Study the drawing (mm; zero at the part's minimum x, y, z) and answer. Give positions to 0.01 mm unless a question says otherwise; leave off trailing zeros. Loops run counter-clockwise (first coordinate to the right, second up) from the corner with the lowest first, then second, coordinate; pieces in that order, holes last. Notation, with made-up numbers: (62.25, 35.25) - (86.25, 35.25) arc R9 ccw to (86.25, 47.25) - close; hole circle Ø4 at (59.5, -0.75). An arc over 180 degrees is marked (long way). Write item = value, one per line. Start each with the question number.
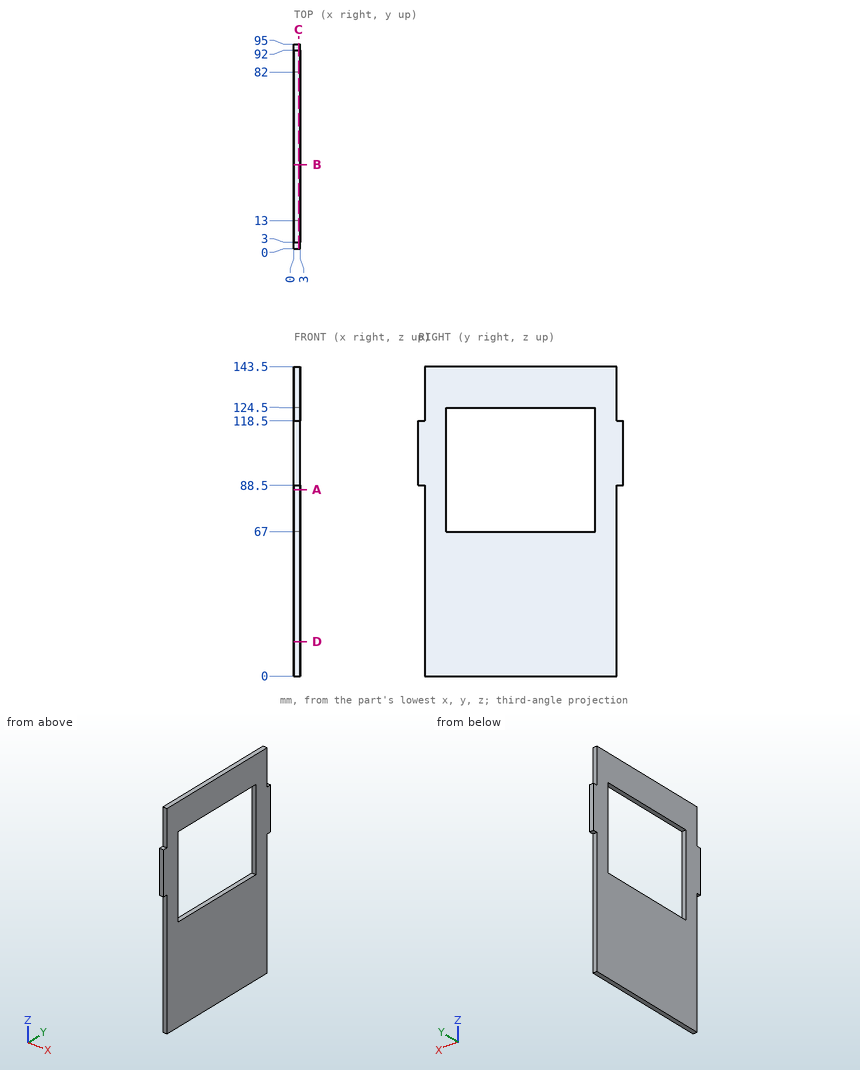
1. A cutting plane is placed at A-A on z = 86.5. Give the vertices of the cut face in (x, y), and give its area (3 significant figures).
2. A cutting plane is placed at D-D on z = 16. Give the vertices of the cut face in (x, y).
3. Consider line 1 along Z through (x, y) = (0.8, 51); line 2 along Y through (x, z) = (2.1, 110.5); line 3 along Y through (x, z) = (2.4, 70.5). Determine where each line is inside the solid, lowest interval first. Write a range as [from, to].
4. A cutting plane is placed at C-C on x = 2.15. Give the vertices of the cut face in (y, z), and give its area (3 significant figures).
5. Given P1, Ø1.5, axis at x = 2, z = 131.5, coming from the +Y side; P2, Ø0.9, axis at x = 2, y = 2, coming from the -Z side; P3, Ø1.5, axis at x = 1, y = 93.5, coming from the +Z side, each flat-ended and moving along its own axis, determine where each tip first touches the part or whether it passes through.
6. A cutting plane is placed at B-B on y = 39. Give the vertices of the cut face in (x, z).
Reply:
q1.outline = (0, 3) - (3, 3) - (3, 13) - (0, 13) - close; (0, 82) - (3, 82) - (3, 92) - (0, 92) - close
q1.area = 60.0 mm^2
q2.outline = (0, 3) - (3, 3) - (3, 92) - (0, 92) - close
q3.line_1 = [0, 67], [124.5, 143.5]
q3.line_2 = [0, 13], [82, 95]
q3.line_3 = [3, 13], [82, 92]
q4.outline = (0, 88.5) - (3, 88.5) - (3, 0) - (92, 0) - (92, 88.5) - (95, 88.5) - (95, 118.5) - (92, 118.5) - (92, 143.5) - (3, 143.5) - (3, 118.5) - (0, 118.5) - close; hole (13, 67) - (82, 67) - (82, 124.5) - (13, 124.5) - close
q4.area = 8,980 mm^2
q5.P1 = 92
q5.P2 = 88.5
q5.P3 = 118.5
q6.outline = (0, 0) - (3, 0) - (3, 67) - (0, 67) - close; (0, 124.5) - (3, 124.5) - (3, 143.5) - (0, 143.5) - close
